```python
from build123d import *

# Parameters (mm, degrees)
SKETCH_1_W          = 120
SKETCH_1_H          = 30
EXTRUDE_2_DEPTH     = 35
SKETCH_1_8_R        = 3
EXTRUDE_3_DEPTH     = 5
SKETCH_2_W          = 40
SKETCH_2_H          = 19.883815918
CUT_EXTRUDE_1_DEPTH = 30


with BuildPart() as part:
    # Sketch 1 → Extrude 2 (new body)
    with BuildSketch(Plane.XY):
        Rectangle(SKETCH_1_W, SKETCH_1_H)
    extrude(amount=EXTRUDE_2_DEPTH)

    # Sketch 1_8 → Extrude 3 (add)
    with BuildSketch(Plane.XY):
        with BuildLine():
            ThreePointArc((90, 15), (105, 0), (90, -15))
            Line((90, -15), (60, -15))
            Line((60, -15), (60, 15))
            Line((60, 15), (90, 15))
        make_face()
        with Locations((90, 0)):
            Circle(SKETCH_1_8_R, mode=Mode.SUBTRACT)
    extrude(amount=EXTRUDE_3_DEPTH)

    # Sketch 2 → Cut-Extrude 1 (cut)
    with BuildSketch(Plane(origin=(0, 0, 0), x_dir=(-1, 0, 0), z_dir=(0, 0, -1))):
        with Locations((30, 0.058092041)):
            Rectangle(SKETCH_2_W, SKETCH_2_H)
    extrude(amount=-CUT_EXTRUDE_1_DEPTH, mode=Mode.SUBTRACT)


solid = part.part
```
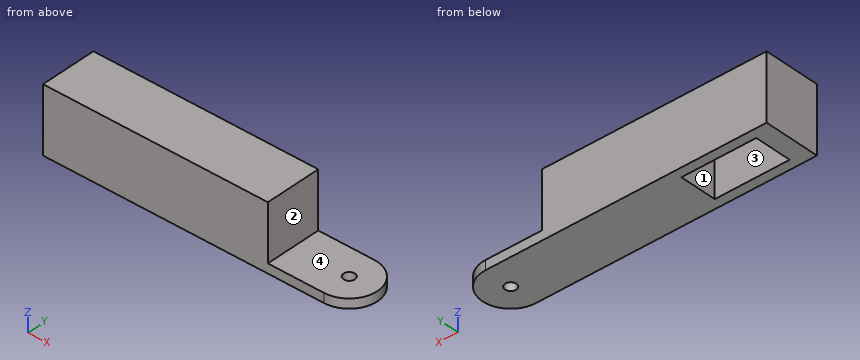
The listing builds one solid part. Answer for the finished solid, in the listing's coordinates (mm). Face numbers are marked on the shaded views. Round coordinates to 2 decimals unless told otherwise and drop trailing zeros. Loops run counter-clockwise (first coordinate to the right, second up) from the corner with the lowest first, then second, coordinate; pieces in that order, holes last.
1) A cutting plane is placed at C-C on z = 9. Determine the outline of the cut face in (x, y).
Outcome:
outline: (-60, -15) - (60, -15) - (60, 15) - (-60, 15) - close; hole (-50, -9.88) - (-10, -9.88) - (-10, 10) - (-50, 10) - close
2) Given P1, Ø9.5, axis at x = 90, y = 0, coming from the -Z side; P2, Ø4, axis at x = -29, y = -3.5, coming from the -Z side; P3, Ø1, axis at y = 8.5, z = 30, coming from the +X side; P4, Ø15, axis at x = 82.5, y = -3.5, coming from the +Z side, each flat-ended and moving along its own axis, determine where each tip first touches the part or whether it passes through.
Outcome:
P1: stops at z = 0
P2: stops at z = 30
P3: stops at x = 60
P4: stops at z = 5
3) A cutting plane is placed at B-B on z = 3. Determine the outline of the cut face in (x, y).
Outcome:
outline: (-60, -15) - (90, -15) arc R15 ccw to (90, 15) - (-60, 15) - close; hole (-50, -9.88) - (-10, -9.88) - (-10, 10) - (-50, 10) - close; hole circle Ø6 at (90, 0)
4) A cutting plane is placed at D-D on x = -12. Determine the outline of the cut face in (y, z), plus the area to 3 significant figures.
Outcome:
outline: (-15, 0) - (-9.88, 0) - (-9.88, 30) - (10, 30) - (10, 0) - (15, 0) - (15, 35) - (-15, 35) - close
area: 453 mm2
5) A cutting plane is placed at A-A on y = 0. Determine the outline of the cut face in (x, z), plus the area to 4 significant figures.
Outcome:
outline: (-60, 0) - (-50, 0) - (-50, 30) - (-10, 30) - (-10, 0) - (87, 0) - (87, 5) - (60, 5) - (60, 35) - (-60, 35) - close; (93, 0) - (105, 0) - (105, 5) - (93, 5) - close
area: 3,195 mm2
6) For a pull along X with two mould halves and no side action, classify the marked faces 1, 2, 3 and 4 as released by +X, released by -X, zero draft, split by the parting line, or undercut.
Outcome:
face 1: undercut
face 2: released by +X
face 3: undercut
face 4: zero draft
7) Consider line 1 (X direction, y = -1.5, z = 15.5); line 2 (Y direction, x = 90, z = 1.8); line 3 (Y direction, x = -31.5, z = 7). Determine where each line is inside the solid, lowest interval first.
Outcome:
line 1: x = -60 to -50, -10 to 60
line 2: y = -15 to -3, 3 to 15
line 3: y = -15 to -9.88, 10 to 15
